```python
from build123d import *

# Parameters (mm, degrees)
SKETCH2_W           = 40
SKETCH2_H           = 30
BOSS_EXTRUDE1_DEPTH = 2
SKETCH3_R           = 4
SKETCH3_R_2         = 2.975
BOSS_EXTRUDE2_DEPTH = 1.35
FILLET1_R           = 1
SKETCH4_R           = 1.5
CUT_EXTRUDE1_DEPTH  = 2


with BuildPart() as part:
    # Sketch2 → Boss-Extrude1 (new body)
    with BuildSketch(Plane(origin=(0, 0, 0), x_dir=(0, 0, -1), z_dir=(1, 0, 0))):
        with Locations((20, 15)):
            Rectangle(SKETCH2_W, SKETCH2_H)
    extrude(amount=BOSS_EXTRUDE1_DEPTH)

    # Sketch3 → Boss-Extrude2 (add)
    # profile 1 of 3: a face of its own
    with BuildSketch(Plane(origin=(2, 0, 0), x_dir=(0, 0, -1), z_dir=(1, 0, 0))):
        with Locations(Location((8.5, 17, 0), (0, 0, 180))):
            Circle(SKETCH3_R)
        with Locations(Location((8.5, 17, 0), (0, 0, 180))):
            Circle(SKETCH3_R_2, mode=Mode.SUBTRACT)
    # profile 2 of 3: a face of its own
    with BuildSketch(Plane(origin=(2, 0, 0), x_dir=(0, 0, -1), z_dir=(1, 0, 0))):
        with Locations(Location((20, 15, 0), (0, 0, 180))):
            Circle(SKETCH3_R)
        with Locations(Location((20, 15, 0), (0, 0, 180))):
            Circle(SKETCH3_R_2, mode=Mode.SUBTRACT)
    # profile 3 of 3: a face of its own
    with BuildSketch(Plane(origin=(2, 0, 0), x_dir=(0, 0, -1), z_dir=(1, 0, 0))):
        with Locations(Location((31.5, 17, 0), (0, 0, 180))):
            Circle(SKETCH3_R)
        with Locations(Location((31.5, 17, 0), (0, 0, 180))):
            Circle(SKETCH3_R_2, mode=Mode.SUBTRACT)
    extrude(amount=BOSS_EXTRUDE2_DEPTH)

    # Fillet1
    fillet1_edges = [part.edges().sort_by_distance(p)[0] for p in [
        (2, 17, -12.5),
        (2, 15, -24),
        (2, 17, -35.5),
    ]]
    fillet(fillet1_edges, radius=FILLET1_R)

    # Sketch4 → Cut-Extrude1 (cut)
    with BuildSketch(Plane.ZY):
        with Locations((-37, 27)):
            Circle(SKETCH4_R)
        with Locations((-3, 27)):
            Circle(SKETCH4_R)
        with Locations((-37, 3)):
            Circle(SKETCH4_R)
        with Locations((-3, 3)):
            Circle(SKETCH4_R)
    extrude(amount=-CUT_EXTRUDE1_DEPTH, mode=Mode.SUBTRACT)


solid = part.part
```
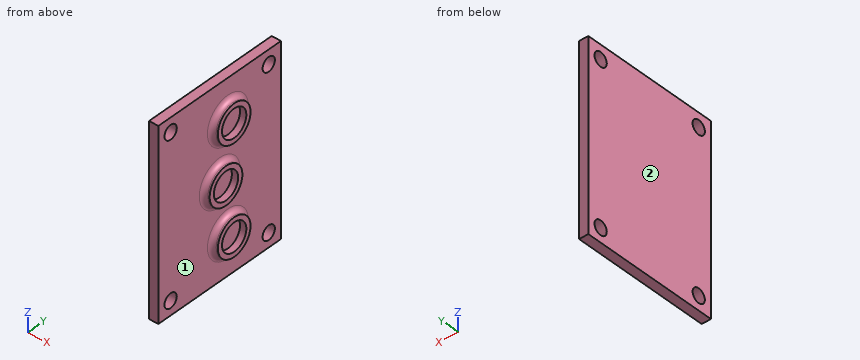
Read the model definition and answer for the solid it produces. Units are mm, in the model's axes. Face numbers are marked on the shaded views. A direction names the side the tool comes from. Coordinates: 2 decimals unless noted, no trailing zeros. Loops run counter-clockwise (first coordinate to the right, second up) from the corner with the lowest first, then second, coordinate; pieces in that order, holes last.
(1) A flat-ended cylindrical pin translates along its axis: pin 1 Ø3 at (y, z) = (16, -30.5) entering from +X. Find the tip coordinate at first contact, or state that the pin passes through.
Solution:
pin 1: stops at x = 2
(2) Consider line 1 along Y through (x, z) = (0.75, -37); line 2 along Z through (x, y) = (2.9, 17) (3 decimals); line 3 along X through (y, z) = (19.25, -37). Determine where each line is inside the solid, lowest interval first.
Solution:
line 1: y = 0 to 1.5, 4.5 to 25.5, 28.5 to 30
line 2: z = -35.505 to -34.475, -28.525 to -27.495, -23.47 to -22.202, -17.798 to -16.53, -12.505 to -11.475, -5.525 to -4.495
line 3: x = 0 to 2
(3) A tool of negligible diameter and unlimited length cuts with its end or side. For the marked faces 1 and 2, from which of +Z, -Z, +X, -X, +Y, -Y can it reach the whole face along a straight path? Write none if from no direction.
Solution:
face 1: +X
face 2: +Z, -Z, -X, +Y, -Y
(4) The part is cut by section C-C (z = -8.5). Determine the outline of the cut face in (x, y) (3 decimals).
Solution:
outline: (0, 0) - (2, 0) - (2, 12) arc R1 cw to (3, 13) - (3.35, 13) - (3.35, 14.025) - (2, 14.025) - (2, 19.975) - (3.35, 19.975) - (3.35, 21) - (3, 21) arc R1 cw to (2, 22) - (2, 30) - (0, 30) - close
(5) The part is cut by section D-D (y = 9.5). Determine the outline of the cut face in (x, z).
Solution:
outline: (0, -40) - (2, -40) - (2, 0) - (0, 0) - close
(6) The part is cut by section B-B (y = 27). Determine the outline of the cut face in (x, z), and give its area (3 significant figures).
Solution:
outline: (0, -40) - (2, -40) - (2, -38.5) - (0, -38.5) - close; (0, -35.5) - (2, -35.5) - (2, -4.5) - (0, -4.5) - close; (0, -1.5) - (2, -1.5) - (2, 0) - (0, 0) - close
area: 68.0 mm2
(7) The part is cut by section A-A (z = -37). Determine the outline of the cut face in (x, y).
Solution:
outline: (0, 0) - (2, 0) - (2, 1.5) - (0, 1.5) - close; (0, 4.5) - (2, 4.5) - (2, 25.5) - (0, 25.5) - close; (0, 28.5) - (2, 28.5) - (2, 30) - (0, 30) - close
